```python
from build123d import *

# Parameters (mm, degrees)
SKETCH_1_R               = 75
EXTRUDE_1_DEPTH          = 30
EXTRUDE_1_TAPER          = 30
CUT_EXTRUDE_1_DEPTH      = 111.227038425
CUT_EXTRUDE_1_DEPTH_BACK = 111.227038425
SKETCH_2_R               = 25
EXTRUDE_2_DEPTH          = 5
FILLET_1_R               = 2.5


with BuildPart() as part:
    # 스케치1 → 보스-돌출1 (new body)
    with BuildSketch(Plane.XY):
        Circle(SKETCH_1_R)
    extrude(amount=EXTRUDE_1_DEPTH, taper=EXTRUDE_1_TAPER)

    # 스케치2 → 컷-돌출1 (cut, two sides: drawn at the far end of the back side and taken through both)
    with BuildSketch(Plane.XY.offset(30).offset(-CUT_EXTRUDE_1_DEPTH_BACK)):
        Circle(SKETCH_2_R)
    extrude(amount=CUT_EXTRUDE_1_DEPTH + CUT_EXTRUDE_1_DEPTH_BACK, mode=Mode.SUBTRACT)

    # 스케치3 → 보스-돌출2 (add)
    with BuildSketch(Plane.XY.offset(30)):
        with BuildLine():
            ThreePointArc((-46.339745962, 0), (-41.339745962, -5), (-36.339745962, 0))
            Line((-36.339745962, 0), (-46.339745962, 0))
        make_face()
        with BuildLine():
            Line((-46.339745962, 0), (-36.339745962, 0))
            ThreePointArc((-36.339745962, 0), (-41.339745962, 5), (-46.339745962, 0))
        make_face()
    extrude(amount=EXTRUDE_2_DEPTH)

    # 필렛1
    fillet_1_edges = [part.edges().sort_by_distance(p)[0] for p in [
        (-46.339745962, 0, 35),
    ]]
    fillet(fillet_1_edges, radius=FILLET_1_R)


solid = part.part
```
Work out the finished part from the listing and answer in its coordinate system (mm). A direction names the side the tool comes from. Give positions to 0.01 mm unless a question says otherwise; leave off trailing zeros. Write each loop counter-clockwise with the first axis right and the second up, starting at its lowest first coordinate (ties: lowest second). Pieces come first, ordered by that corner, then holes.
(1) The part is cut by section A-A on x = 0. Write down the section's boundary in (y, z).
Final values:
outline: (-75, 0) - (-25, 0) - (-25, 30) - (-57.68, 30) - close; (25, 0) - (75, 0) - (57.68, 30) - (25, 30) - close
(2) Straight lines are drawn through the part: line 1 (Z direction, x = -44, y = -10); line 2 (X direction, y = -8, z = 1); line 3 (X direction, y = 9.5, z = 19). For each, find the intervals that lie inside material, in ascending order.
Final values:
line 1: z = 0 to 30
line 2: x = -73.99 to -23.69, 23.69 to 73.99
line 3: x = -63.32 to -23.12, 23.12 to 63.32
(3) The part is cut by section B-B on z = 23. Write down the section's boundary in (x, y).
Final values:
outline: circle Ø123.44 at (0, 0); hole circle Ø50 at (0, 0)
(4) The part is cut by section C-C on z = 4. Write down the section's boundary in (x, y), plus the area to 3 significant figures.
Final values:
outline: circle Ø145.38 at (0, 0); hole circle Ø50 at (0, 0)
area: 14,600 mm2
(5) The mould has two halves that part along X. Classify faces 1 (the conical face through (-7.618, 58.023, 28.543)), 2 (the flat face through (-18, 18, 0)), 3 (the cylindrical face through (23.846, 7.509, 14.79)): pulls with the +X half, pulls with the -X half, needs draft (parallel to the pull), parting line crosses it, or undercut.
Final values:
face 1: parting line crosses it
face 2: needs draft
face 3: undercut
(6) Which of the six approach directions +Z, -Z, +X, -X, +Y, -Y give full straight-line access (tool end or side, diameter ignored) to faces 4 (the cylindrical face through (-36.721, -1.915, 31.232)), 5 (the flat face through (-41, 0, 35))?
Final values:
face 4: +Z
face 5: +Z, +X, -X, +Y, -Y
(7) Flat-ended cylindrical pins translate along their axes: pin 1 Ø12 at (y, z) = (-26, 22.5) entering from +X; pin 2 Ø5 at (x, z) = (-47, 25.5) entering from -Y; pin 3 Ø8 at (x, z) = (2.5, 13) entering from -Y. Find the tip coordinate at first contact, or state that the pin passes through.
Final values:
pin 1: stops at x = 60.81
pin 2: stops at y = -41.4
pin 3: stops at y = -69.76
